```python
from build123d import *

# Parameters (mm, degrees)
F1_DEPTH  = 10
F3_W      = 10
F3_H      = 30
F6_W      = 80
F6_H      = 30
F7_DEPTH  = 5
F8_R      = 3.25
F9_DEPTH  = 5
F10_W     = 9
F10_H     = 3
F11_DEPTH = 100


with BuildPart() as f1:
    # F0 (on Top) → F1 (new body)
    with BuildSketch(Plane.XY):
        Polygon((-52.5, 43.769281), (-57, 0), (-44, 0), (-42.5, 43.769281), align=None)
        Polygon((42.5, 43.769281), (44, 0), (57, 0), (52.5, 43.769281), align=None)
    extrude(amount=F1_DEPTH)

    # F1_face (on face) → F4 section 0
    with BuildSketch(Plane(origin=(-49.065217, 20.933135, 10), x_dir=(1, 0, 0), z_dir=(0, 0, 1))):
        Polygon((-3.434783, 22.836147), (-7.934783, -20.933135), (5.065217, -20.933135), (6.565217, 22.836147), align=None)
    # F3 (on offset) → F4 section 1
    with BuildSketch(Plane.XY.offset(40)):
        with Locations((-35, 15)):
            Rectangle(F3_W, F3_H)
    loft()

    # F1_face (on face) → F5 section 0
    with BuildSketch(Plane(origin=(-49.065217, 20.933135, 10), x_dir=(1, 0, 0), z_dir=(0, 0, 1))):
        Polygon((91.565217, 22.836147), (93.065217, -20.933135), (106.065217, -20.933135), (101.565217, 22.836147), align=None)
    # F3 (on offset) → F5 section 1
    with BuildSketch(Plane.XY.offset(40)):
        with Locations((35, 15)):
            Rectangle(F3_W, F3_H)
    loft()

    # F6 (on offset) → F7 (join)
    with BuildSketch(Plane.XY.offset(40)):
        with Locations((0, 15)):
            Rectangle(F6_W, F6_H)
    extrude(amount=-F7_DEPTH)

    # F8 (on offset) → F9 (cut, through all)
    with BuildSketch(Plane.XY.offset(40)):
        with Locations((0, 5)):
            Circle(F8_R)
    extrude(amount=-F9_DEPTH, mode=Mode.SUBTRACT)

    # F10 (on Right) → F11 (cut, symmetric)
    with BuildSketch(Plane.YZ):
        with Locations((10.5, 4.5)):
            Rectangle(F10_W, F10_H)
        with Locations((33.269281, 4.5)):
            Rectangle(F10_W, F10_H)
    extrude(amount=F11_DEPTH, both=True, mode=Mode.SUBTRACT)


solid = f1.part
```
Check sheet for the modelled part. Datum: model origin and axes. Units: mm. A direction names the side the tool comes from. Give positions to 0.01 mm unless a question says otherwise; leave off trailing zeros. Loops run counter-clockwise (first coordinate to the right, second up) from the corner with the lowest first, then second, coordinate; pieces in that order, holes last. Notation, with made-up numbers: M 1.25,-5.75 L 6.25,-5.75 A14 ccw 6.25,14.25 Z; hole C 73,18.5 d3. An arc over 180 degrees is marked long. Answer in a Markdown table with one row per item.
1) Cross-section at B-B (y = 10.5). Count the separate pieces of the cut face and the enclosed holes in it, plus the area to 3 significant figures.
Solutions:
| item | result |
|---|---|
| separate pieces | 3 |
| enclosed holes | 0 |
| area | 1,150 mm^2 |
2) Tool access check on faces 4 (the face through (-54.72, 22.19, 4.93)), 5 (the face through (0, 15, 35)), 6 (the face through (48, 37.769, 4)). Record the directions out of +Z, -Z, +X, -X, +Y, -Y that give a thin tool (end or side, any length) a straight path to the whole face; none if there is none.
Solutions:
| item | result |
|---|---|
| face 4 | +Z, -Z, -X, +Y |
| face 5 | -Z, +Y, -Y |
| face 6 | +X, -X |
3) Depth check by flat-ended pin: pin 1 (10 mm diameter, centred on y = 16.5, z = 14, fed in from -X); pin 2 (3 mm diameter, centred on x = -34.5, y = 15, fed in from -Z); pin 3 (2 mm diameter, centred on x = 30, y = 26.5, fed in from -Z). Enter the tip coordinate at first touch or a pass-through.
Solutions:
| item | result |
|---|---|
| pin 1 | stops at x = -55.61 |
| pin 2 | stops at z = 26.54 |
| pin 3 | stops at z = 35 |
4) Cross-section at C-C (x = -17). Enter the section's corners in (y, z).
Solutions:
| item | result |
|---|---|
| outline | M 0,35 L 30,35 L 30,40 L 0,40 Z |
5) Mould release check, pull along Z, two halves, no side actions. Record for faces 1 (the face through (-50, 10, 3)), 2 (the face through (54.78, 21.58, 4.93)), 3 (the face through (50, 22, 0)): released by +Z, released by -Z, zero draft, split by the parting line, or undercut.
Solutions:
| item | result |
|---|---|
| face 1 | undercut |
| face 2 | zero draft |
| face 3 | released by -Z |
6) Cross-section at A-A (x = 0). Enter the section's corners in (y, z).
Solutions:
| item | result |
|---|---|
| outline | M 0,35 L 1.75,35 L 1.75,40 L 0,40 Z; M 8.25,35 L 30,35 L 30,40 L 8.25,40 Z |
7) Thickness scan on line 1 (Y direction, x = 0, z = 37.55); line 2 (Z direction, x = 29, y = 17); line 3 (Z direction, x = -46, y = 35.5). Record the ranges inside material, lowest first.
Solutions:
| item | result |
|---|---|
| line 1 | y = 0 to 1.75, 8.25 to 30 |
| line 2 | z = 35 to 40 |
| line 3 | z = 0 to 3, 6 to 25.75 |
